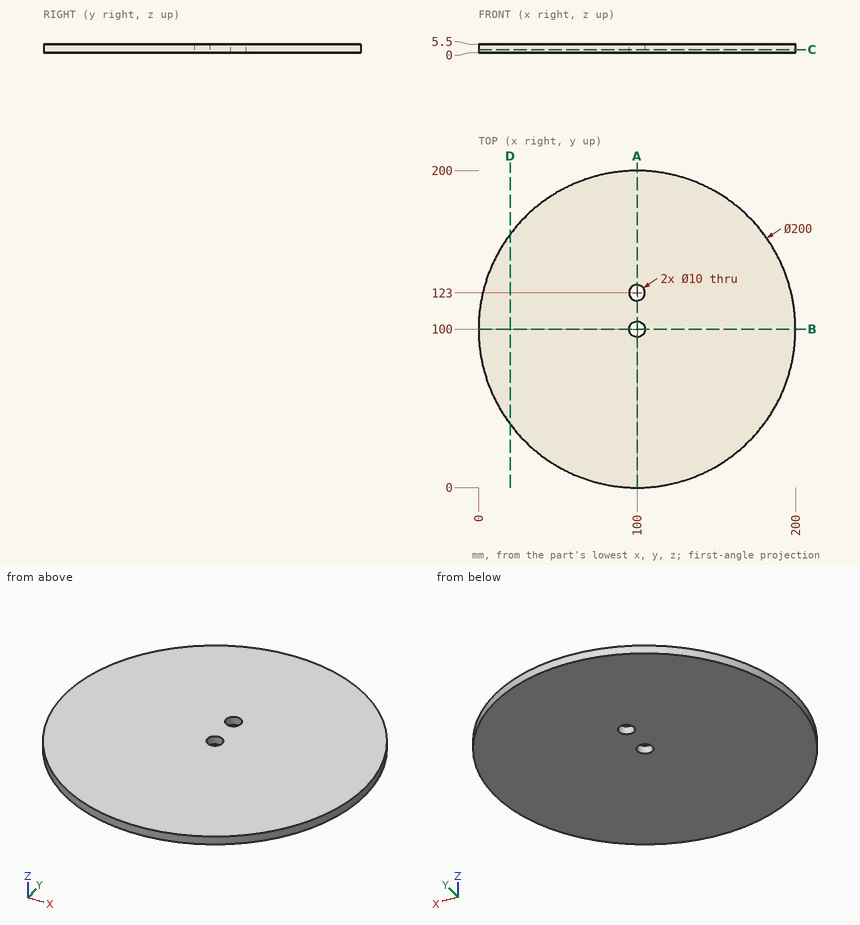
For this review, use the dimensioned drawing (mm, ordinates from the lowest corner) and the shaded views. Coordinates: 2 decimals unless noted, no trailing zeros. Write each loop counter-clockwise with the first axis right and the second up, starting at its lowest first coordinate (ties: lowest second). Pieces come first, ordered by that corner, then holes. Notation, with made-up numbers: (40.25, -12.75) - (87.25, -12.75) arc R22 ccw to (87.25, -3.75) - close; hole circle Ø2 at (68, -13.75). An arc over 180 degrees is marked (long way). Answer in a Markdown table with one row per item. Add a question column.
Q1. Consider section D-D on x = 20. Give the boundary of the cut face in (y, z).
Q2. Clearance check with flat-ended pins moving along their axes: pin 1 (1.5 mm diameter, centred on x = 20.5, z = 1.5, fed in from +Y); pin 2 (6 mm diameter, centred on x = 100, y = 100, fed in from -Z); pin 3 (1 mm diameter, centred on x = 72.5, z = 4.5, fed in from +Y). State where each tip first meets the part, or that it passes through.
Q3. Consider section C-C on z = 2. Give the boundary of the cut face in (x, y).
Q4. Consider section B-B on y = 100. Give the boundary of the cut face in (x, z), then the cut area to 4 significant figures.
Q5. To check wall thickness, follow line 1 along Y through (x, z) = (100, 2.9); line 2 along X through (y, z) = (119.5, 2.9); line 3 along Y through (x, z) = (117.5, 0.8). State the ranges of each line that lie inside material, in increasing order. Write a range as from..to.
Q6. Consider section A-A on x = 100. Give the boundary of the cut face in (y, z).
Answers below:
| question | item | result |
|---|---|---|
| 1 | outline | (40, 0) - (160, 0) - (160, 5.5) - (40, 5.5) - close |
| 2 | pin 1 | y = 161.63 |
| 2 | pin 2 | through |
| 2 | pin 3 | y = 196.29 |
| 3 | outline | circle Ø200 at (100, 100); hole circle Ø10 at (100, 100); hole circle Ø10 at (100, 123) |
| 4 | outline | (0, 0) - (95, 0) - (95, 5.5) - (0, 5.5) - close; (105, 0) - (200, 0) - (200, 5.5) - (105, 5.5) - close |
| 4 | area | 1,045 mm² |
| 5 | line 1 | 0..95, 105..118, 128..200 |
| 5 | line 2 | 1.92..96.43, 103.57..198.08 |
| 5 | line 3 | 1.54..198.46 |
| 6 | outline | (0, 0) - (95, 0) - (95, 5.5) - (0, 5.5) - close; (105, 0) - (118, 0) - (118, 5.5) - (105, 5.5) - close; (128, 0) - (200, 0) - (200, 5.5) - (128, 5.5) - close |
